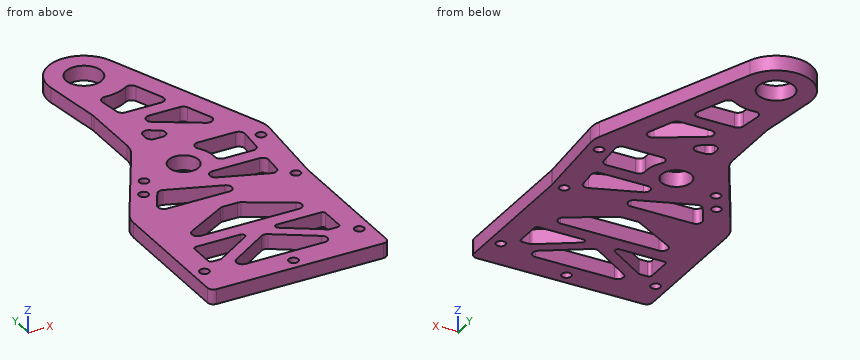
```python
from build123d import *

# Parameters (mm, degrees)
SKETCH_1_R          = 6
SKETCH_1_R_2        = 1.6
SKETCH_1_R_3        = 5
EXTRUDE_1_DEPTH     = 5
FILLET_1_R          = 2
FILLET_2_R          = 10
CUT_EXTRUDE_1_DEPTH = 146.740914343
FILLET_3_R          = 2
FILLET_4_R          = 1
FILLET_5_R          = 2
FILLET_7_R          = 2
SKETCH_4_R          = 1.6
CUT_EXTRUDE_2_DEPTH = 146.740914343


with BuildPart() as part:
    # 草图1 → 凸台-拉伸1 (new body)
    with BuildSketch(Plane.XY):
        with BuildLine():
            Line((-30, 0), (30, 0))
            Line((30, 0), (30, 49))
            Line((30, 49), (32.588678263, 78.58872794))
            Line((32.588678263, 78.58872794), (11.202965118, 134.300415395))
            ThreePointArc((11.202965118, 134.300415395), (-2.951546295, 141.63135308), (-11.897955052, 128.438377258))
            Line((-11.897955052, 128.438377258), (-9.215390309, 108))
            Line((-9.215390309, 108), (-9.215390309, 85))
            Line((-9.215390309, 85), (-30, 49))
            Line((-30, 49), (-30, 0))
        make_face()
        with Locations((0, 130)):
            Circle(SKETCH_1_R, mode=Mode.SUBTRACT)
        with Locations((0, 4)):
            Circle(SKETCH_1_R_2, mode=Mode.SUBTRACT)
        with Locations((26, 11)):
            Circle(SKETCH_1_R_2, mode=Mode.SUBTRACT)
        with Locations((-26, 11)):
            Circle(SKETCH_1_R_2, mode=Mode.SUBTRACT)
        with Locations((0, 70)):
            Circle(SKETCH_1_R_3, mode=Mode.SUBTRACT)
        with Locations((-15.196152423, 66.641016151)):
            Circle(SKETCH_1_R_2, mode=Mode.SUBTRACT)
        with Locations((-19.196152423, 59.712812921)):
            Circle(SKETCH_1_R_2, mode=Mode.SUBTRACT)
    extrude(amount=EXTRUDE_1_DEPTH)

    # 圆角1
    fillet_1_edges = [part.edges().sort_by_distance(p)[0] for p in [
        (30, 0, 2.5),
        (-30, 0, 2.5),
    ]]
    fillet(fillet_1_edges, radius=FILLET_1_R)

    # 圆角2
    # the kernel refuses this fillet: 10 mm, written as the material it adds along each edge
    with BuildSketch(Plane(origin=(-9.215390309, 85, 0), x_dir=(-0.5000000000000011, -0.8660254037844379, 0), z_dir=(0, 0, 1))) as fillet_2_piece_1:
        with BuildLine():
            CenterArc((FILLET_2_R * 0.267949192431, -FILLET_2_R), FILLET_2_R, 90, 30)
            Line((-FILLET_2_R * 0.232050807569, -FILLET_2_R * 0.133974596216), (0, 0))
            Line((0, 0), (FILLET_2_R * 0.267949192431, 0))
        make_face()
    extrude(amount=5)
    with BuildSketch(Plane(origin=(-9.215390309, 108, 0), x_dir=(0, -1, 0), z_dir=(0, 0, 1))) as fillet_2_piece_2:
        with BuildLine():
            CenterArc((FILLET_2_R * 0.0653454548024, -FILLET_2_R), FILLET_2_R, 90, 7.47740672)
            Line((-FILLET_2_R * 0.0647897736728, -FILLET_2_R * 0.00850374569053), (0, 0))
            Line((0, 0), (FILLET_2_R * 0.0653454548024, 0))
        make_face()
    extrude(amount=5)
    with BuildSketch(Plane(origin=(30, 49, 0), x_dir=(0, -1, 0), z_dir=(0, 0, 1))) as fillet_2_piece_3:
        with BuildLine():
            CenterArc((FILLET_2_R * 0.0436609429085, FILLET_2_R), FILLET_2_R, 265, 5)
            Line((-FILLET_2_R * 0.0434947998391, FILLET_2_R * 0.00380530190825), (0, 0))
            Line((0, 0), (FILLET_2_R * 0.0436609429085, 0))
        make_face()
    extrude(amount=5)
    # the kernel refuses this fillet: 10 mm, written as the material it takes off along each edge
    with BuildSketch(Plane(origin=(-30, 49, -6.698729811), x_dir=(0, -1, 0), z_dir=(0, 0, 1))) as fillet_2_2_piece_1:
        with BuildLine():
            CenterArc((FILLET_2_R * 0.267949192431, FILLET_2_R), FILLET_2_R, 240, 30)
            Line((-FILLET_2_R * 0.232050807569, FILLET_2_R * 0.133974596216), (0, 0))
            Line((0, 0), (FILLET_2_R * 0.267949192431, 0))
        make_face()
    extrude(amount=18.397459622, mode=Mode.SUBTRACT)
    with BuildSketch(Plane(origin=(32.588678263, 78.58872794, -5.771704778), x_dir=(-0.08715574274765964, -0.9961946980917453, 0), z_dir=(0, 0, 1))) as fillet_2_2_piece_2:
        with BuildLine():
            CenterArc((FILLET_2_R * 0.230868191126, -FILLET_2_R), FILLET_2_R, 90, 26)
            Line((-FILLET_2_R * 0.207502955664, -FILLET_2_R * 0.101205953701), (0, 0))
            Line((0, 0), (FILLET_2_R * 0.230868191126, 0))
        make_face()
    extrude(amount=16.543409556, mode=Mode.SUBTRACT)

    # 草图3 → 切除-拉伸1 (cut, through all)
    with BuildSketch(Plane(origin=(0, 0, 0), x_dir=(-1, 0, 0), z_dir=(0, 0, -1))):
        Polygon((-20, 9), (20, 9), (0, 22), align=None)
        Polygon((-22, 15), (-18.108837195, 15), (-2.72422181, 25), (-22, 25), align=None)
        Polygon((22, 25), (22, 15), (18.108837195, 15), (2.72422181, 25), align=None)
        Polygon((-24, 30), (-3, 30), (3, 30), (24, 30), (3, 42), (-3, 42), align=None)
        Polygon((-14.748572851, 49), (20.762395693, 49), (14.525138112, 59.80324703), align=None)
        Polygon((6.035973745, 62), (-23.106793925, 62), (-22.195289828, 51.581460488), align=None)
        with BuildLine():
            Line((-23.544237243, 67), (-9.539392014, 67))
            ThreePointArc((-9.539392014, 67), (-9.180992478, 73.96350566), (-4.358898944, 79))
            Line((-4.358898944, 79), (-24.594101205, 79))
            Line((-24.594101205, 79), (-23.544237243, 67))
        make_face()
        with BuildLine():
            Line((1.761599482, 105), (-14.952325844, 105))
            Line((-14.952325844, 105), (-9.354171163, 119.583691543))
            ThreePointArc((-9.354171163, 119.583691543), (-3.443470677, 116.430088073), (3.255742342, 116.383827931))
            Line((3.255742342, 116.383827931), (1.761599482, 105))
        make_face()
        Polygon((-16.871646019, 100), (2.128353981, 100), (-22.629606545, 85), align=None)
        Polygon((2.215390309, 94.206636856), (-9.679385078, 87), (2.215390309, 87), align=None)
    extrude(amount=-CUT_EXTRUDE_1_DEPTH, mode=Mode.SUBTRACT)

    # 圆角3
    fillet_3_edges = [part.edges().sort_by_distance(p)[0] for p in [
        (20, 9, 2.5),
        (0, 22, 2.5),
        (-20, 9, 2.5),
    ]]
    fillet(fillet_3_edges, radius=FILLET_3_R)

    # 圆角4
    fillet_4_edges = [part.edges().sort_by_distance(p)[0] for p in [
        (-2.72422181, 25, 2.5),
        (-22, 25, 2.5),
        (-22, 15, 2.5),
        (-18.108837195, 15, 2.5),
        (22, 15, 2.5),
        (22, 25, 2.5),
        (2.72422181, 25, 2.5),
        (18.108837195, 15, 2.5),
    ]]
    fillet(fillet_4_edges, radius=FILLET_4_R)

    # 圆角5
    fillet_5_edges = [part.edges().sort_by_distance(p)[0] for p in [
        (23.544237243, 67, 2.5),
        (24.594101205, 79, 2.5),
        (4.358898944, 79, 2.5),
        (9.539392014, 67, 2.5),
        (22.195289828, 51.581460488, 2.5),
        (23.106793925, 62, 2.5),
        (-6.035973745, 62, 2.5),
        (-14.525138112, 59.80324703, 2.5),
        (-20.762395693, 49, 2.5),
        (14.748572851, 49, 2.5),
        (24, 30, 2.5),
        (3, 42, 2.5),
        (-3, 42, 2.5),
        (-24, 30, 2.5),
    ]]
    fillet(fillet_5_edges, radius=FILLET_5_R)

    # 圆角7
    fillet_7_edges = [part.edges().sort_by_distance(p)[0] for p in [
        (-3.255742342, 116.383827931, 2.5),
        (-1.761599482, 105, 2.5),
        (14.952325844, 105, 2.5),
        (9.354171163, 119.583691543, 2.5),
        (22.629606545, 85, 2.5),
        (16.871646019, 100, 2.5),
        (-2.128353981, 100, 2.5),
        (-2.215390309, 94.206636856, 2.5),
        (-2.215390309, 87, 2.5),
        (9.679385078, 87, 2.5),
    ]]
    fillet(fillet_7_edges, radius=FILLET_7_R)

    # 草图4 → 切除-拉伸2 (cut, through all)
    with BuildSketch(Plane(origin=(0, 0, 0), x_dir=(-1, 0, 0), z_dir=(0, 0, -1))):
        with Locations((-25.993043669, 49.095132548)):
            Circle(SKETCH_4_R)
        with Locations((-28.171937238, 74)):
            Circle(SKETCH_4_R)
    extrude(amount=-CUT_EXTRUDE_2_DEPTH, mode=Mode.SUBTRACT)


solid = part.part
```
CAD build for the part. Positions are in the model's coordinates, mm. Round coordinates to 2 decimals unless told otherwise and drop trailing zeros. Loops run counter-clockwise (first coordinate to the right, second up) from the corner with the lowest first, then second, coordinate; pieces in that order, holes last. Notation, with made-up numbers: M 24,71.25 L 60,71.25 A35 ccw 60,109.25 Z; hole C 29,65.5 d3. An arc over 180 degrees is marked long. Return JSON: item names as keys, results as strings. Group by question number.
(1) Wall check: probe 1 along X at (y, z) = (67.5, 4.3); probe 2 along Y at (x, z) = (-5.5, 2.95) (3 decimals); probe 3 along X at (y, z) = (10.5, 3.2). Give the ranges that are in metal, low to high. Write a range as [from, to].
(2) Saw through at B-B, the plane x = -26. List the corners of the cut face in (y, z).
(3) Drop flat-ended pins along their axis: P1, Ø11, axis at x = 0, y = 130, coming from the -Z side; P2, Ø2.5, axis at x = -1.5, z = 3, coming from the +Y side; P3, Ø2.5, axis at y = 20, z = 2, coming from the +X side; P4, Ø4, axis at x = -26, y = 11, coming from the -Z side. Give the stop position or say it passes through.
(4) Saw through at A-A, the plane y = 35.5. List the corners of the cut face in (x, z) (3 decimals), and give its area (3 significant figures).
(5) Saw through at C-C, the plane z = 3.95. Give the number of separate pieces and of enclosed holes in the cut face, and give its area (3 significant figures).
Answer list:
{
 "1": {"probe 1": "[-19.32, -16.55], [-13.85, -4.33], [4.33, 10.64], [23.03, 31.62]", "probe 2": "[0, 9], [18.425, 23.198], [24.802, 30], [40.571, 49], [56.473, 127.602], [132.398, 140.665]", "probe 3": "[-30, -27.52], [-24.48, -15.19], [15.19, 24.48], [27.52, 30]"},
 "2": {"outline": "M 0,0 L 9.4,0 L 9.4,5 L 0,5 Z; M 12.6,0 L 55.93,0 L 55.93,5 L 12.6,5 Z"},
 "3": {"P1": "through", "P2": "y = 142", "P3": "x = 30", "P4": "z = 0"},
 "4": {"outline": "M -30,0 L -14.375,0 L -14.375,5 L -30,5 Z; M 14.375,0 L 30,0 L 30,5 L 14.375,5 Z", "area": "156 mm2"},
 "5": {"separate pieces": "1", "enclosed holes": "19", "area": "4,580 mm2"}
}
